Check sheet for the drawn part. Datum: minimum x, y, z corner. Units: mm. A direction names the side the tool comes from. Give positions to 0.01 mm unless a question says otherwise; leave off trailing zeros. Loops run counter-clockwise (first coordinate to the right, second up) from the corner with the lowest first, then second, coordinate; pieces in that order, holes last.
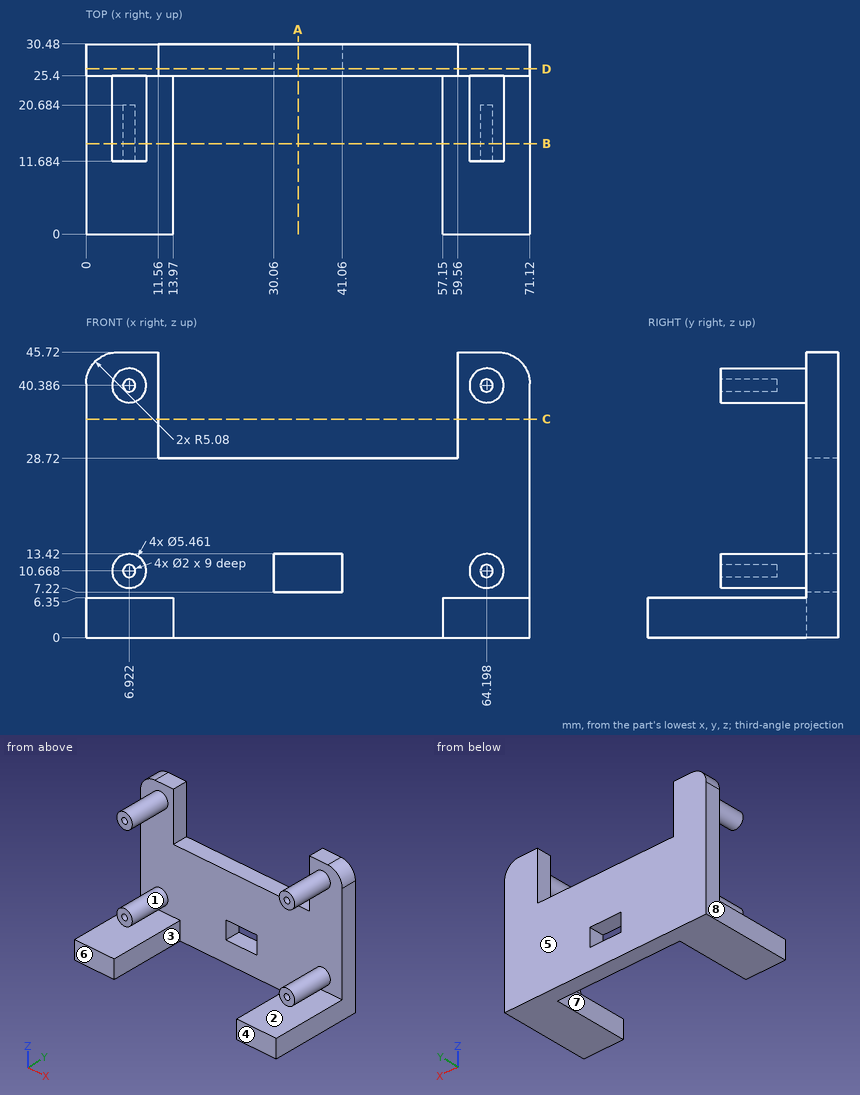
1) Depth check by flat-ended pin: P1, Ø15.5, axis at x = 65, y = 15, coming from the +Z side; P2, Ø1, axis at x = 7.5, z = 10.5, coming from the -Y side; P3, Ø5, axis at x = 57, y = 23.5, coming from the +Z side. Enter the tip coordinate at first touch or a pass-through.
2) Sectioned sample at B-B on y = 14.5. Count the separate pieces of the cut face and the enclosed holes in it.
3) Mould release check, pull along X, two halves, no side actions. Record for the marked faces 6, 7 and 8: +X half, -X half, draft (parallel to the pull), parting line (faces both ways), or undercut.
4) Sectioned sample at D-D on y = 26.5. Enter the section's corners in (x, z), plus the area to 3 significant figures.
5) Scan lines: line 1 along X through (y, z) = (28, 8.5); line 2 along X through (y, z) = (8.5, 3); line 3 along Y through (x, z) = (8.5, 36.5). Record each from-to range of solid material in increasing order.
6) Tool access check on the marked faces 1, 2, 3, 4 and 5. Record the directions out of +Z, -Z, +X, -X, +Y, -Y that give a thin tool (end or side, any length) a straight path to the whole face; none if there is none.
7) Sectioned sample at C-C on z = 35. Enter the section's corners in (x, y).
8) Sectioned sample at A-A on x = 34. Enter the section's corners in (y, z).
Determined:
1. P1: stops at z = 43.12
1. P2: stops at y = 11.68
1. P3: stops at z = 28.72
2. separate pieces: 6
2. enclosed holes: 4
3. face 6: draft
3. face 7: undercut
3. face 8: -X half
4. outline: (0, 0) - (71.12, 0) - (71.12, 40.64) arc R5.08 ccw to (66.04, 45.72) - (59.56, 45.72) - (59.56, 28.72) - (11.56, 28.72) - (11.56, 45.72) - (5.08, 45.72) arc R5.08 ccw to (0, 40.64) - close; hole (30.06, 7.22) - (41.06, 7.22) - (41.06, 13.42) - (30.06, 13.42) - close
4. area: 2,360 mm2
5. line 1: x = 0 to 30.06, 41.06 to 71.12
5. line 2: x = 0 to 13.97, 57.15 to 71.12
5. line 3: y = 25.4 to 30.48
6. face 1: -Y
6. face 2: +X, -X, -Y
6. face 3: +Z, -Z, -Y
6. face 4: +Z, -Z, +X, -X, -Y
6. face 5: +Z, -Z, +X, -X, +Y
7. outline: (0, 25.4) - (11.56, 25.4) - (11.56, 30.48) - (0, 30.48) - close; (59.56, 25.4) - (71.12, 25.4) - (71.12, 30.48) - (59.56, 30.48) - close
8. outline: (25.4, 0) - (30.48, 0) - (30.48, 7.22) - (25.4, 7.22) - close; (25.4, 13.42) - (30.48, 13.42) - (30.48, 28.72) - (25.4, 28.72) - close
